from build123d import *

# Parameters (mm, degrees)
SKETCH1_W               = 38.1
SKETCH1_H               = 12.7
BOSS_EXTRUDE1_DEPTH     = 376.2
SKETCH2_R               = 6.35
CUT_EXTRUDE1_DEPTH      = 1
CUT_EXTRUDE1_DEPTH_BACK = 13.7


with BuildPart() as part:
    # Sketch1 → Boss-Extrude1 (new body)
    with BuildSketch(Plane(origin=(0, 0, 0), x_dir=(0, 0, -1), z_dir=(1, 0, 0))):
        with Locations((19.05, 6.35)):
            Rectangle(SKETCH1_W, SKETCH1_H)
    extrude(amount=BOSS_EXTRUDE1_DEPTH)

    # Sketch2 → Cut-Extrude1 (cut, two sides)
    with BuildSketch(Plane(origin=(0, 12.7, 0), x_dir=(1, 0, 0), z_dir=(0, 1, 0))) as cut_extrude1_sk:
        with Locations((308.1, 23)):
            Circle(SKETCH2_R)
        with Locations((228.1, 23)):
            Circle(SKETCH2_R)
        with Locations((148.1, 23)):
            Circle(SKETCH2_R)
        with Locations((68.1, 23)):
            Circle(SKETCH2_R)
    extrude(amount=CUT_EXTRUDE1_DEPTH, mode=Mode.SUBTRACT)
    extrude(cut_extrude1_sk.sketch, amount=-CUT_EXTRUDE1_DEPTH_BACK, mode=Mode.SUBTRACT)


solid = part.part
Part model, mm, in its own coordinate system. Coordinates: 2 decimals unless noted, no trailing zeros. Loops run counter-clockwise (first coordinate to the right, second up) from the corner with the lowest first, then second, coordinate; pieces in that order, holes last. Notation, with made-up numbers: M 36.25,-9.75 L 71.25,-9.75 A8 ccw 71.25,4.25 Z; hole C 4.25,40 d10. An arc over 180 degrees is marked long. Use a Markdown table: item, result. Add a question column.
Q1. Cut at A-A (z = -23). Write the cut outline in (x, y), and give its area (3 significant figures).
Q2. Cut at C-C (x = 228.1). Write the cut outline in (y, z).
Q3. Mould opens along Z. For faces 1 (the flat face through (185, 6, -38.1)), 2 (the cylindrical face through (74.157, 6.439, -24.907)), 3 (the flat face through (185, 12.7, -19)) say: +Z half, -Z half, draft (parallel to the pull), parting line (faces both ways), or undercut.
Q4. Cut at B-B (y = 7). Write the cut outline in (x, z), and give its area (3 significant figures).
Q5. Probe L1, parallel to X at y = 5, z = -23; L2, parallel to Z at x = 68.1, y = 5.25. List the from-to ranges inside material, lowest first.
Worked out:
| question | item | result |
|---|---|---|
| 1 | outline | M 0,0 L 61.75,0 L 61.75,12.7 L 0,12.7 Z; M 74.45,0 L 141.75,0 L 141.75,12.7 L 74.45,12.7 Z; M 154.45,0 L 221.75,0 L 221.75,12.7 L 154.45,12.7 Z; M 234.45,0 L 301.75,0 L 301.75,12.7 L 234.45,12.7 Z; M 314.45,0 L 376.2,0 L 376.2,12.7 L 314.45,12.7 Z |
| 1 | area | 4,130 mm2 |
| 2 | outline | M 0,-38.1 L 12.7,-38.1 L 12.7,-29.35 L 0,-29.35 Z; M 0,-16.65 L 12.7,-16.65 L 12.7,0 L 0,0 Z |
| 3 | face 1 | -Z half |
| 3 | face 2 | undercut |
| 3 | face 3 | draft |
| 4 | outline | M 0,-38.1 L 376.2,-38.1 L 376.2,0 L 0,0 Z; hole C 68.1,-23 d12.7; hole C 148.1,-23 d12.7; hole C 228.1,-23 d12.7; hole C 308.1,-23 d12.7 |
| 4 | area | 13,800 mm2 |
| 5 | L1 | x = 0 to 61.75, 74.45 to 141.75, 154.45 to 221.75, 234.45 to 301.75, 314.45 to 376.2 |
| 5 | L2 | z = -38.1 to -29.35, -16.65 to 0 |
